Check sheet for the modelled part. Datum: model origin and axes. Units: mm. A direction names the side the tool comes from. Coordinates: 2 decimals unless noted, no trailing zeros. Loops run counter-clockwise (first coordinate to the right, second up) from the corner with the lowest first, then second, coordinate; pieces in that order, holes last. Notation, with made-up numbers: (50.5, -27) - (108.5, -27) arc R5 ccw to (108.5, -22) - close; hole circle Ø8 at (29.5, -20.5). An arc over 180 degrees is marked (long way). Use a Markdown table: item, result. Add a question column.
1) Go/stop test with flat-tipped pins: P1, Ø1.5, axis at x = -3, y = 45.5, coming from the -Z side; P2, Ø4, axis at x = -49.5, z = -14.5, coming from the +Y side; P3, Ø10, axis at x = 5.5, z = -19, coming from the +Y side. Record where each tip stops, or that it passes through.
2) Sectioned sample at B-B, the plane z = -25. Enter the section's corners in (x, y) (3 decimals), then the cut area to 3 significant figures.
3) Sectioned sample at C-C, the plane y = 3. Enter the section's corners in (x, z), then the cut area to 3 significant figures.
4) Sectioned sample at D-D, the plane z = -3.5. Enter the section's corners in (x, y).
5) Tool access check on faces 1 (the flat face through (-62.93, 35, -16)), 2 (the flat face through (24, 39.375, -21)), 3 (the flat face through (-24.73, -24, -21)), 4 (the flat face through (23, 62.125, -21)), 5 (the flat face through (-22.73, -23, -22)). Record the directions out of +Z, -Z, +X, -X, +Y, -Y that give a thin tool (end or side, any length) a straight path to the whole face; none if there is none.
6) Draft check along Y on faces 6 (the cylindrical face through (24.185, 52.022, 1.217)), 7 (the flat face through (-32, 45, 0)), 8 (the flat face through (0.02, -24, -22)), 9 (the flat face through (23, 41.375, -22)). Enter one of: pulls with the +Y half, pulls with the -Y half, needs draft (parallel to the pull), parting line crosses it, or undercut.
7) Thickness scan on line 1 (Y direction, x = 34, z = -24.5) (3 decimals); line 2 (X direction, y = -23, z = -15.5); line 3 (X direction, y = 21.5, z = -18). Record the ranges inside material, lowest first.
8) Sectioned sample at A-A, the plane x = -38.5. Enter the section's corners in (y, z), then the cut area to 3 significant figures.
from build123d import *

# Parameters (mm, degrees)
F1_DEPTH  = 32
F3_DEPTH  = 2
F5_DEPTH  = 2
F7_DEPTH  = 2
F9_DEPTH  = 45
F11_DEPTH = 45


with BuildPart() as f1:
    # F0 (on Top) → F1 (new body)
    with BuildSketch(Plane.XY):
        Polygon((2, 71.536247), (-16.671573, 90.20782), (-46.258427, 90.20782), (-64.93, 71.536247), (-64.93, -2), (2, -2), align=None)
        Polygon((0, 70.70782), (0, 0), (-62.93, 0), (-62.93, 70.70782), (-45.43, 88.20782), (-17.5, 88.20782), align=None, mode=Mode.SUBTRACT)
    extrude(amount=-F1_DEPTH)

    # F2 (on face) → F3 (join)
    with BuildSketch(Plane.XY):
        Polygon((-64.93, 71.536247), (-64.93, -2), (2, -2), (2, 71.536247), (-16.671573, 90.20782), (-46.258427, 90.20782), align=None)
    extrude(amount=F3_DEPTH)

    # F4 (on face) → F5 (cut)
    with BuildSketch(Plane.XZ.offset(2)):
        with BuildLine():
            ThreePointArc((-12.355, -0.78), (-19.691233, -3.818767), (-22.73, -11.155))
            Line((-22.73, -11.155), (-22.73, -32))
            Line((-22.73, -32), (-1.98, -32))
            Line((-1.98, -32), (-1.98, -11.155))
            ThreePointArc((-1.98, -11.155), (-5.018767, -3.818767), (-12.355, -0.78))
        make_face()
    extrude(amount=-F5_DEPTH, mode=Mode.SUBTRACT)

    # F6 (on face) → F7 (cut)
    with BuildSketch(Plane.YZ.offset(2)):
        with BuildLine():
            Line((62.125, -32), (62.125, -11.155))
            ThreePointArc((62.125, -11.155), (59.086233, -3.818767), (51.75, -0.78))
            ThreePointArc((51.75, -0.78), (44.413767, -3.818767), (41.375, -11.155))
            Line((41.375, -11.155), (41.375, -32))
            Line((41.375, -32), (62.125, -32))
        make_face()
    extrude(amount=-F7_DEPTH, mode=Mode.SUBTRACT)

    # F8 (on face) → F9 (join)
    with BuildSketch(Plane.XZ.offset(2)):
        with BuildLine():
            ThreePointArc((0.02, -11.155), (-12.355, 1.22), (-24.73, -11.155))
            Line((-24.73, -11.155), (-24.73, -32))
            Line((-24.73, -32), (-22.73, -32))
            Line((-22.73, -32), (-22.73, -11.155))
            ThreePointArc((-22.73, -11.155), (-12.355, -0.78), (-1.98, -11.155))
            Line((-1.98, -11.155), (-1.98, -32))
            Line((-1.98, -32), (0.02, -32))
            Line((0.02, -32), (0.02, -11.155))
        make_face()
    extrude(amount=F9_DEPTH)

    # F10 (on face) → F11 (join)
    with BuildSketch(Plane.YZ.offset(2)):
        with BuildLine():
            ThreePointArc((64.125, -11.155), (51.75, 1.22), (39.375, -11.155))
            Line((39.375, -11.155), (39.375, -32))
            Line((39.375, -32), (41.375, -32))
            Line((41.375, -32), (41.375, -11.155))
            ThreePointArc((41.375, -11.155), (51.75, -0.78), (62.125, -11.155))
            Line((62.125, -11.155), (62.125, -32))
            Line((62.125, -32), (64.125, -32))
            Line((64.125, -32), (64.125, -11.155))
        make_face()
    extrude(amount=F11_DEPTH)


solid = f1.part
Solved:
| question | item | result |
|---|---|---|
| 1 | P1 | stops at z = 0 |
| 1 | P2 | stops at y = 88.97 |
| 1 | P3 | stops at y = 73.04 |
| 2 | outline | (-64.93, -2) - (-24.73, -2) - (-24.73, -47) - (-22.73, -47) - (-22.73, 0) - (-62.93, 0) - (-62.93, 70.708) - (-45.43, 88.208) - (-17.5, 88.208) - (0, 70.708) - (0, 62.125) - (47, 62.125) - (47, 64.125) - (2, 64.125) - (2, 71.536) - (-16.672, 90.208) - (-46.258, 90.208) - (-64.93, 71.536) - close; (-1.98, -47) - (0.02, -47) - (0.02, -2) - (2, -2) - (2, 39.375) - (47, 39.375) - (47, 41.375) - (0, 41.375) - (0, 0) - (-1.98, 0) - close |
| 2 | area | 855 mm2 |
| 3 | outline | (-64.93, -32) - (-62.93, -32) - (-62.93, 0) - (0, 0) - (0, -32) - (2, -32) - (2, 2) - (-64.93, 2) - close |
| 3 | area | 262 mm2 |
| 4 | outline | (-64.93, -2) - (-22.08, -2) - (-22.08, -47) - (-19.36, -47) - (-19.36, 0) - (-62.93, 0) - (-62.93, 70.71) - (-45.43, 88.21) - (-17.5, 88.21) - (0, 70.71) - (0, 58.75) - (47, 58.75) - (47, 61.47) - (2, 61.47) - (2, 71.54) - (-16.67, 90.21) - (-46.26, 90.21) - (-64.93, 71.54) - close; (-5.35, -47) - (-2.63, -47) - (-2.63, -2) - (2, -2) - (2, 42.03) - (47, 42.03) - (47, 44.75) - (0, 44.75) - (0, 0) - (-5.35, 0) - close |
| 5 | face 1 | -Z |
| 5 | face 2 | +Z, -Z, +X, -Y |
| 5 | face 3 | +Z, -Z, -X, -Y |
| 5 | face 4 | -Z, +X |
| 5 | face 5 | -Z, -Y |
| 6 | face 6 | parting line crosses it |
| 6 | face 7 | undercut |
| 6 | face 8 | needs draft |
| 6 | face 9 | undercut |
| 7 | line 1 | y = 39.375 to 41.375, 62.125 to 64.125 |
| 7 | line 2 | x = -24.73 to -22.73, -1.98 to 0.02 |
| 7 | line 3 | x = -64.93 to -62.93, 0 to 2 |
| 8 | outline | (-2, -32) - (0, -32) - (0, 0) - (88.21, 0) - (88.21, -32) - (90.21, -32) - (90.21, 2) - (-2, 2) - close |
| 8 | area | 312 mm2 |
